Verification items for the finished model (mm, model axes). Coordinates: 2 decimals unless noted, no trailing zeros. Loops run counter-clockwise (first coordinate to the right, second up) from the corner with the lowest first, then second, coordinate; pieces in that order, holes last. Notation, with made-up numbers: (-2.75, 9.25) - (37.25, 9.25) arc R26 cw to (37.25, 45.25) - close; hole circle Ø5 at (-27, 74). An arc over 180 degrees is marked (long way). One line per item, written item: value. Start each with the question number.
(1) Section check A-A (y = 1.2). Record the boundary of the cut face in (x, z) (3 decimals), plus the area to 3 significant figures.
(2) Section check B-B (z = 50.5). Record the boundary of the cut face in (x, y) (3 decimals), plus the area to 3 significant figures.
(3) Thickness scan on probe 1 along Z at (x, y) = (-87.5, 2.4) (3 decimals); probe 2 along Z at (x, y) = (-80, 2.85) (3 decimals); probe 3 along X at (y, z) = (1.55, -49.5). Record the ranges inside material, lowest first. Write a range as [from, to].
(4) Section check C-C (x = -80). Record the boundary of the cut face in (y, z) (3 decimals), plus the area to 3 significant figures.
(5) Gauge pin test, flat end, axial feed: P1, Ø1, axis at x = -69, y = 1.5, coming from the +Z side. Record the tip position at first contact, or that the pin passes through.
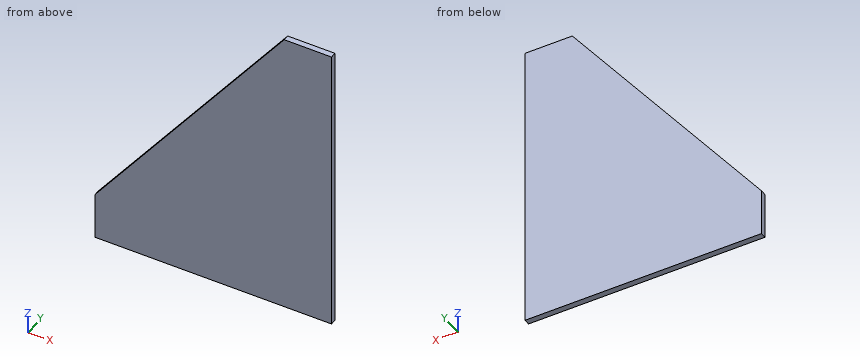
```python
from build123d import *

# Parameters (mm, degrees)
SKETCH1_W           = 101.6
SKETCH1_H           = 25.4
SKETCH1_W_2         = 25.4
SKETCH1_H_2         = 158.75
BOSS_EXTRUDE1_DEPTH = 3.175


with BuildPart() as part:
    # Sketch1 → Boss-Extrude1 (new body)
    with BuildSketch(Plane(origin=(0, 0, 0), x_dir=(1, 0, 0), z_dir=(0, 1, 0))):
        with Locations((-63.5, 66.675)):
            Rectangle(SKETCH1_W, SKETCH1_H)
        Polygon((-12.7, -79.375), (-12.7, 53.975), (-114.3, 53.975), align=None)
        Rectangle(SKETCH1_W_2, SKETCH1_H_2)
    extrude(amount=BOSS_EXTRUDE1_DEPTH)


solid = part.part
```
Responses:
1. outline: (-114.3, -79.375) - (12.7, -79.375) - (12.7, 79.375) - (-12.7, 79.375) - (-114.3, -53.975) - close
1. area: 13,400 mm²
2. outline: (-34.7, 0) - (12.7, 0) - (12.7, 3.175) - (-34.7, 3.175) - close
2. area: 150 mm²
3. probe 1: z = [-79.375, -18.8]
3. probe 2: z = [-79.375, -8.956]
3. probe 3: x = [-110.89, 12.7]
4. outline: (0, -79.375) - (3.175, -79.375) - (3.175, -8.956) - (0, -8.956) - close
4. area: 224 mm²
5. P1: stops at z = 6.14
